For this review, take the finished solid that the model builds, in its own axes (mm). A direction names the side the tool comes from. Round coordinates to 2 decimals unless told otherwise and drop trailing zeros. Write each loop counter-clockwise with the first axis right and the second up, starting at its lowest first coordinate (ties: lowest second). Pieces come first, ordered by that corner, then holes.
from build123d import *

# Parameters (mm, degrees)
F0_W     = 100
F0_H     = 200
F1_DEPTH = 800
F2_R     = 10
F3_DEPTH = 10
F4_R     = 10
F5_DEPTH = 100


with BuildPart() as f1:
    # F0 (on Front) → F1 (new body)
    with BuildSketch(Plane.XZ):
        with Locations((-50, 100)):
            Rectangle(F0_W, F0_H)
    extrude(amount=F1_DEPTH)

    # F2 (on face) → F3 (cut)
    with BuildSketch(Plane.YZ):
        with Locations((-750, 150)):
            Circle(F2_R)
        with Locations((-750, 50)):
            Circle(F2_R)
        with Locations((-50, 150)):
            Circle(F2_R)
        with Locations((-50, 50)):
            Circle(F2_R)
    extrude(amount=-F3_DEPTH, mode=Mode.SUBTRACT)

    # F4 (on face) → F5 (cut)
    with BuildSketch(Plane.XY.offset(200)):
        with Locations((-50, -250)):
            Circle(F4_R)
        with Locations((-50, -540)):
            Circle(F4_R)
    extrude(amount=-F5_DEPTH, mode=Mode.SUBTRACT)


solid = f1.part
(1) For line 1 along Z through (x, y) = (-6.5, -750); line 2 along Y through (x, z) = (-50, 162); line 3 along X through (y, z) = (-246, 147), list the stretches that pass through material, from the lowest coordinate up.
Geometry check:
line 1: z = 0 to 40, 60 to 140, 160 to 200
line 2: y = -800 to -550, -530 to -260, -240 to 0
line 3: x = -100 to -59.17, -40.83 to 0
(2) Mouldability with a two-part tool opening along Y and no side actions: class faces 4 (the face through (-50, -250, 100)), 5 (the face through (-51, -394, 200)), 6 (the face through (-51, -800, 101)) as pulls with the +Y half, pulls with the -Y half, needs draft (parallel to the pull), parting line crosses it, or undercut.
Geometry check:
face 4: undercut
face 5: needs draft
face 6: pulls with the -Y half
(3) We need section C-C, the plane y = -540. Give the boundary of the cut face in (x, z).
Geometry check:
outline: (-100, 0) - (0, 0) - (0, 200) - (-40, 200) - (-40, 100) - (-60, 100) - (-60, 200) - (-100, 200) - close
(4) We need section A-A, the plane y = -50. Give the boundary of the cut face in (x, z).
Geometry check:
outline: (-100, 0) - (0, 0) - (0, 40) - (-10, 40) - (-10, 60) - (0, 60) - (0, 140) - (-10, 140) - (-10, 160) - (0, 160) - (0, 200) - (-100, 200) - close
(5) For faces 1 (the face through (-10, -50, 50)), 2 (the face through (-51.302, -530.085, 150.7)), 3 (the face through (-100, -394, 99)), list the 3-axis set-ups (+Z, -Z, +X, -X, +Y, -Y) from which the entire face can be reached by the end or side of a thin tool; tool diameter is ignored.
Geometry check:
face 1: +X
face 2: +Z
face 3: +Z, -Z, -X, +Y, -Y
(6) We need section B-B, the plane x = -50. Give the boundary of the cut face in (y, z), and give its area (3 significant figures).
Geometry check:
outline: (-800, 0) - (0, 0) - (0, 200) - (-240, 200) - (-240, 100) - (-260, 100) - (-260, 200) - (-530, 200) - (-530, 100) - (-550, 100) - (-550, 200) - (-800, 200) - close
area: 156,000 mm2
(7) For pin 1 Ø12 at (x, y) = (-15, -400) entering from -Z; pin 2 Ø6 at (x, y) = (-54.5, -251.5) entering from +Z; pin 3 Ø18 at (y, z) = (-750, 50) entering from +X, all flat-tipped, find the tip position at first contact; note any pin that passes through.
Geometry check:
pin 1: stops at z = 0
pin 2: stops at z = 100
pin 3: stops at x = -10
